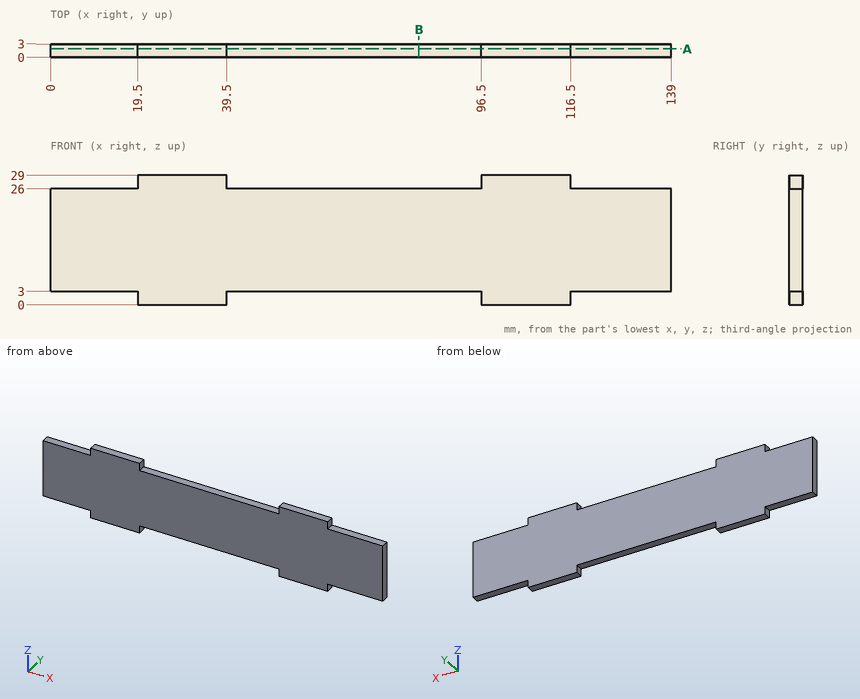
Verification items for this drawing (mm, ordinates from the low corner). Coordinates: 2 decimals unless noted, no trailing zeros. Loops run counter-clockwise (first coordinate to the right, second up) from the corner with the lowest first, then second, coordinate; pieces in that order, holes last.
Item 1: Go/stop test with flat-tipped pins: pin 1 Ø0.9 at (x, y) = (128, 2) entering from +Z; pin 2 Ø1.5 at (y, z) = (2, 2) entering from +X; pin 3 Ø1.5 at (x, y) = (13, 1.5) entering from -Z. Record where each tip stops, or that it passes through.
Item 2: Sectioned sample at A-A, the plane y = 1.9. Record the boundary of the cut face in (x, z), then the cut area to 3 significant figures.
Item 3: Sectioned sample at B-B, the plane x = 82.5. Record the boundary of the cut face in (y, z).
Item 4: Thickness scan on line 1 (X direction, y = 0.75, z = 27.25); line 2 (Z direction, x = 65.5, y = 2.75). Record the ranges inside material, lowest first.
Check result:
1. pin 1: stops at z = 26
1. pin 2: stops at x = 116.5
1. pin 3: stops at z = 3
2. outline: (0, 3) - (19.5, 3) - (19.5, 0) - (39.5, 0) - (39.5, 3) - (96.5, 3) - (96.5, 0) - (116.5, 0) - (116.5, 3) - (139, 3) - (139, 26) - (116.5, 26) - (116.5, 29) - (96.5, 29) - (96.5, 26) - (39.5, 26) - (39.5, 29) - (19.5, 29) - (19.5, 26) - (0, 26) - close
2. area: 3,440 mm2
3. outline: (0, 3) - (3, 3) - (3, 26) - (0, 26) - close
4. line 1: x = 19.5 to 39.5, 96.5 to 116.5
4. line 2: z = 3 to 26
